CAD build for the part. Positions are in the model's coordinates, mm. A direction names the side the tool comes from. Give positions to 0.01 mm unless a question says otherwise; leave off trailing zeros. Order: outer loops, then holes, each group sorted by start corner. A loop starts at its lowest first (then second) coordinate and runs counter-clockwise, first axis right, second up.
Item 1: Band-saw the part on A-A on z = 0. Give the cut face in (x, y), plus the area to 3 significant figures.
Item 2: Band-saw the part on C-C on y = 1. Give the cut face in (x, z).
Item 3: Flat gauge pins, fed straight in: P1, Ø0.7, axis at y = 1.5, z = 1.5, coming from the +X side; P2, Ø3, axis at x = -0.5, z = -6, coming from the -Y side; P3, Ø0.5, axis at x = 0.5, z = -1.5, coming from the -Y side. Where does each tip first touch, or does it go through?
Item 4: Wall check: L1, parallel to X at y = 0.05, z = 0; L2, parallel to Z at x = 0, y = 0.9; L3, parallel to X at y = 1, z = -1.25. Give the ranges that are in metal, low to high.
Item 5: Which spindle directions (+Z, -Z, +X, -X, +Y, -Y) get a long thin tool onto all of the face, cutting with end or side? Do faces 1 (the flat face through (-1, 1, 2)), 2 (the cylindrical face through (1.742, -1.737, 1.085)). Say none if no direction does.
Item 6: Band-saw the part on D-D on z = -1.5. Give the cut face in (x, y).
Item 7: Band-saw the part on B-B on x = 0. Give the cut face in (y, z) (3 decimals), plus the area to 3 significant figures.
```python
from build123d import *

# Parameters (mm, degrees)
BOSS_EXTRUDE1_DEPTH      = 2.5
CUT_EXTRUDE8_DEPTH       = 5.330127019
CUT_EXTRUDE8_DEPTH_BACK  = 5.330127019
BOSS_EXTRUDE2_REACH      = 14.744
BOSS_EXTRUDE2_END_RADIUS = 2.5
SKETCH6_R                = 1.125
BOSS_EXTRUDE4_REACH      = 20.144
BOSS_EXTRUDE4_START      = -5.4
SKETCH7_R                = 1.375
SKETCH5_R                = 0.125


with BuildPart() as part:
    # Sketch3 → Boss-Extrude1 (new, symmetric)
    with BuildSketch(Plane(origin=(0, 0, 0), x_dir=(1, 0, 0), z_dir=(0, 1, 0))):
        with BuildLine():
            Line((-1, -1.436140662), (-1, -2.291287847))
            ThreePointArc((-1, -2.291287847), (0, 2.5), (1, -2.291287847))
            Line((1, -2.291287847), (1, -1.436140662))
            ThreePointArc((1, -1.436140662), (0, 1.75), (-1, -1.436140662))
        make_face()
    extrude(amount=BOSS_EXTRUDE1_DEPTH, both=True)

    # Sketch4 → Cut-Extrude8 (cut, two sides: drawn at the far end of the back side and taken through both)
    with BuildSketch(Plane(origin=(0, 0, 0), x_dir=(0, 0, -1), z_dir=(1, 0, 0)).offset(-CUT_EXTRUDE8_DEPTH_BACK)):
        with BuildLine():
            ThreePointArc((-2.291287847, 0.85), (-1.448230481, -1.382297021), (0.66, -2.5))
            Line((0.66, -2.5), (-2.291287847, -2.5))
            Line((-2.291287847, -2.5), (-2.291287847, 0.85))
        make_face()
    extrude(amount=CUT_EXTRUDE8_DEPTH + CUT_EXTRUDE8_DEPTH_BACK, mode=Mode.SUBTRACT)

    # Boss-Extrude2: up to this cylinder (the profile starts outside it)
    boss_extrude2_end = Plane(origin=(0, -2.616609, 0), z_dir=(0, -1, 0)) * Cylinder(BOSS_EXTRUDE2_END_RADIUS, 35.488, mode=Mode.PRIVATE)
    # Sketch6 → Boss-Extrude2 (add, up to the surface)
    with BuildSketch(Plane(origin=(0, -2.616608772, -9.11), x_dir=(-1, 0, 0), z_dir=(0, -0.22222922625140035, -0.9749944466506996)), mode=Mode.PRIVATE) as boss_extrude2_sk1:
        with Locations(Location((0, 0, 0), (0, 0, 90))):
            Circle(SKETCH6_R)
    boss_extrude2_tool1 = extrude(boss_extrude2_sk1.sketch, amount=-BOSS_EXTRUDE2_REACH, mode=Mode.PRIVATE) - boss_extrude2_end
    add(boss_extrude2_tool1.solids().sort_by_distance((0, -2.616609, -9.11))[0])

    # Sketch7 → Boss-Extrude4 (add, up to next)
    with BuildSketch(Plane(origin=(0, -2.616608772, -9.11), x_dir=(-1, 0, 0), z_dir=(0, -0.22222922625140035, -0.9749944466506996)).offset(BOSS_EXTRUDE4_START), mode=Mode.PRIVATE) as boss_extrude4_sk1:
        with Locations(Location((0, 0, 0), (0, 0, 90))):
            Circle(SKETCH7_R)
    boss_extrude4_tool1 = extrude(boss_extrude4_sk1.sketch, amount=-BOSS_EXTRUDE4_REACH, mode=Mode.PRIVATE) - part.part
    add(boss_extrude4_tool1.solids().sort_by_distance((0, -1.416571, -3.84503))[0])

    # Sketch5 → Revolve1 (revolve)
    with BuildSketch(Plane(origin=(0, 0, 0), x_dir=(0, 0, -1), z_dir=(1, 0, 0)), mode=Mode.PRIVATE) as revolve1_sk:
        with Locations((5.11, -2.853618424)):
            Circle(SKETCH5_R)
    revolve(revolve1_sk.sketch.rotate(Axis((0, -1.11, -2.5), (0, -0.22222922625140032, -0.9749944466506997)), 180), axis=Axis((0, -1.11, -2.5), (0, -0.22222922625140032, -0.9749944466506997)))


solid = part.part
```
The answers:
1. outline: (-2.5, -2.35) - (-1.75, -2.35) - (-1.75, 2.5) - (-2.5, 2.5) - close; (1.75, -2.35) - (2.5, -2.35) - (2.5, 2.5) - (1.75, 2.5) - close
1. area: 7.27 mm2
2. outline: (-1, 1.44) - (-1, 2.29) arc R2.5 ccw (long way) to (1, 2.29) - (1, 1.44) arc R1.75 cw (long way) to start
3. P1: stops at x = 2.22
3. P2: stops at y = -3.39
3. P3: stops at y = -2.5
4. L1: x = -2.5 to -1.75, 1.75 to 2.5
4. L2: z = -2.5 to -1.75
4. L3: x = -2.17 to -1.22, 1.22 to 2.17
5. face 1: +Z, +Y, -Y
5. face 2: +Z, +X, -X, -Y
6. outline: (-2, -2.5) - (-0.9, -2.5) - (-0.9, 2.5) - (-2, 2.5) - close; (0.9, -2.5) - (2, -2.5) - (2, 2.5) - (0.9, 2.5) - close
7. outline: (-3.713, -8.86) - (-1.52, -9.36) - (-0.693, -5.731) arc R0.125 ccw to (-0.637, -5.487) - (-0.32, -4.095) - (-0.076, -4.151) - (0.3, -2.5) - (2.5, -2.5) - (2.5, -1.75) - (-2.5, -1.75) - (-2.5, -2.411) - (-2.757, -3.539) - (-2.513, -3.595) - (-2.831, -4.987) arc R0.125 ccw to (-2.886, -5.231) - close
7. area: 19.7 mm2
